Could you check a few things on this model? Use its own coordinates, in mm. Round coordinates to 2 decimals unless told otherwise and drop trailing zeros. Write each loop counter-clockwise with the first axis right and the second up, starting at its lowest first coordinate (ties: lowest second). Pieces come first, ordered by that corner, then holes. Notation, with made-up numbers: M -16,15 L 21,15 A22 ccw 21,34 Z; hole C 32.5,48.25 d4. An arc over 180 degrees is marked long. One line per item, written item: value. Start each with the question number.
(1) If I drill on L1, parallel to Y at x = 24, z = 1.35; L2, parallel to X at y = -45, z = 0.3; L3, parallel to X at y = -21.59, z = 1.25, over which ranges is the centre line in solid material (lowest first)?
(2) I'm going to push a flat-ended pin straight in: pin 1 Ø3 at (x, y) = (20, -47) entering from +Z. Where does the tip first touch, or does it pass through?
(3) Thinking about a two-plate mould opening in X: for faces 1 (the face through (37.3, -51.39, 0.78)), 2 (the face through (-33.027, -62.545, 0.805)), 3 (the face through (12, -40, 1.588)), 4 (the face through (-30.72, -19.87, 0.8)), which applies, released by +X, released by -X, zero draft, split by the parting line, or undercut?
(4) I want a section at A-A on z = 1. Count the separate pieces of the cut face and the enclosed holes in it, and give its area (3 significant figures).
(5) I want a section at C-C on y = -34.29. Please give me the cut outline in (x, z), and give its area (3 significant figures).
(6) I want a section at B-B on x = 41.5. Please give me the cut outline in (y, z).
(7) I want a section at D-D on y = -48.5. Please give me the cut outline in (x, z).
Autodesk Inventor part; units mm, degrees
ref_plane "YZ Plane" through (0, 0, 0) normal (1, 0, 0) x (0, 1, 0)
ref_plane "XZ Plane" through (0, 0, 0) normal (0, 1, 0) x (-1, 0, 0)
ref_plane "XY Plane" through (0, 0, 0) normal (0, 0, 1) x (1, 0, 0)
sketch "Sketch1" plane through (0, 0, 0) normal (0, 0, 1) x (1, 0, 0)
  circle A0 centre (0, 0) radius 63.5
  line L0 (0, 0) -> (63.5, 0)
  line L1 (0, 0) -> (0, -63.5)
  line L2 (0, 0) -> (-127, 0)
  line L3 (-127, 0) -> (-127, -63.5)
  line L4 (-127, -63.5) -> (0, -63.5)
  line L5 (-127, 0) -> (-127, -16.51)
  line L6 (-127, -16.51) -> (61.3161, -16.51)
  dimension "d0" = 127
  dimension "d1" = 127
  dimension "d43" = 16.51
extrude "Extrusion4" add sketch "Sketch1" along normal blind 1.5875 contours L1 L6 A0 | L4 L3 L6 A0 | A0 L6 L1
sketch "Sketch4" plane through (0, 0, 1.5875) normal (0, 0, 1) x (1, 0, 0)
  arc A0 (0, -63.5) -> (61.3161, -16.51) centre (0, 0) ccw
  line L0 (61.3161, -16.51) -> (-59.3339, -16.51)
  line L1 (61.3161, -16.51) -> (-127, -16.51)
  line L2 (-59.3339, -16.51) -> (-59.3339, -62.6422)
  line L3 (-59.3339, -62.6422) -> (-59.3339, -63.5)
  line L4 (-127, -63.5) -> (0, -63.5)
  line L5 (-136.3806, -11.9346) -> (-59.3339, -11.9346)
  line L6 (-59.3339, -11.9346) -> (-59.3339, -68.0966)
  line L7 (-59.3339, -68.0966) -> (-136.3806, -68.0966)
  line L8 (-136.3806, -68.0966) -> (-136.3806, -11.9346)
  point P0 (-59.3339, -16.51)
  dimension "d46" = 120.65
extrude "Extrusion5" cut sketch "Sketch4" against normal blind 1.5875 contours L6 L7 L8 L5 L2 L3
fillet "Fillet2" radius 3.175 1 edges at (61.3161, -16.51, 0.7937)
fillet "Fillet3" radius 3.175 1 edges at (-59.3339, -16.51, 0.7937)
sketch "Sketch5" plane through (0, 0, 1.5875) normal (0, 0, 1) x (1, 0, 0)
  circle A0 centre (-55.6881, -20.1151) radius 2.54
  line L0 (-55.6881, -20.1151) -> (-55.6881, -45.5151)
  line L1 (-55.6881, -45.5151) -> (-55.6881, -58.2151)
  circle A1 centre (-55.6881, -58.2151) radius 2.54
  line L2 (-55.6881, -20.1151) -> (-30.2881, -20.1151)
  line L3 (-55.6881, -58.2151) -> (-30.2881, -58.2151)
  circle A2 centre (-55.6881, -45.5151) radius 2.54
  circle A3 centre (-55.6881, -32.8151) radius 2.54
  line L4 (-59.3339, -13.3218) -> (-33.9321, -13.3218)
  line L5 (-33.9321, -13.3218) -> (-33.9321, -67.3178)
  line L6 (-33.9321, -67.3178) -> (-59.3339, -67.3178)
  line L7 (-59.3339, -67.3178) -> (-59.3339, -13.3218)
  point P0 (0, 0)
  point P1 (-4.8881, -58.2151)
  point P2 (7.8119, -58.2151)
  point P3 (-59.3339, -20.1151)
  point P4 (-42.9881, -20.1151)
  point P5 (-42.9881, -58.2151)
  dimension "d51" = 5.08
  dimension "d52" = 25.4
  dimension "d53" = 12.7
  dimension "d54" = 5.08
  dimension "d55" = 25.4
  dimension "d63" = 25.4
  dimension "d68" = 5.08
  dimension "d69" = 5.08
extrude "Extrusion6" cut sketch "Sketch5" against normal blind 1.5875
sketch "Sketch6" plane through (0, 0, 1.5875) normal (0, 0, 1) x (1, 0, 0)
  line L0 (57.0229, -16.51) -> (-33.9321, -16.51)
  line L1 (-33.9321, -63.5) -> (-33.9321, -16.51)
  line L2 (-33.9321, -21.59) -> (-33.9321, -26.67)
  line L3 (-33.9321, -21.59) -> (-28.8521, -21.59)
  line L4 (-28.8521, -21.59) -> (-28.8521, -16.51)
  circle A0 centre (-28.8521, -21.59) radius 2.54
  line L5 (-28.8521, -21.59) -> (-28.8521, -46.99)
  line L6 (-28.8521, -46.99) -> (-28.8521, -59.69)
  circle A1 centre (-28.8521, -59.69) radius 2.54
  line L7 (-28.8521, -21.59) -> (-3.4521, -21.59)
  line L8 (-3.4521, -21.59) -> (21.9479, -21.59)
  line L9 (21.9479, -21.59) -> (47.3479, -21.59)
  circle A2 centre (-28.8521, -34.29) radius 2.54
  circle A3 centre (-28.8521, -46.99) radius 2.54
  line L10 (-28.8521, -59.69) -> (-3.4521, -59.69)
  line L11 (-3.4521, -59.69) -> (9.2479, -59.69)
  circle A4 centre (47.3479, -21.59) radius 2.54
  line L12 (21.9479, -34.29) -> (21.9479, -46.99)
  circle A5 centre (21.9479, -34.29) radius 2.54
  circle A6 centre (21.9479, -46.99) radius 2.54
  line L13 (21.9479, -34.29) -> (42.2679, -34.29)
  circle A7 centre (42.2679, -34.29) radius 2.54
  line L14 (21.9479, -34.29) -> (33.3071, -44.45)
  circle A8 centre (33.3071, -44.45) radius 2.54
  point P0 (0, 0)
  dimension "d80" = 5.08
  dimension "d81" = 5.08
  dimension "d82" = 5.08
  dimension "d83" = 25.4
  dimension "d84" = 12.7
  dimension "d85" = 5.08
  dimension "d86" = 25.4
  dimension "d87" = 25.4
  dimension "d88" = 25.4
  dimension "d89" = 5.08
  dimension "d90" = 5.08
  dimension "d91" = 25.4
  dimension "d92" = 12.7
  dimension "d96" = 5.08
  dimension "d99" = 5.08
  dimension "d100" = 5.08
  dimension "d101" = 5.08
  dimension "d102" = 20.32
  dimension "d103" = 15.24
  dimension "d104" = 5.08
extrude "Extrusion7" cut sketch "Sketch6" against normal blind 5.08 contours A4 | A1 L10 L6 | L6 L10 A1 | A3 L6 L5 | L5 L6 A3 | A2 L5 | L5 A2 | A0 L7 L4 | L4 L3 A0 | L5 A0 L3 | L7 A0 L5 | L14 A5 L12 | L12 A5 L13 | L13 A5 L14 | A6 | A7 | A8
fillet "Fillet4" radius 3.175 2 edges at (-33.9321, -16.51, 0.7937) (-33.9321, -63.5, 0.7937)
equation "\"d97\" = d93"
properties part number "Sleds"
Found:
1. L1: y = -58.79 to -48.49, -45.49 to -35.79, -32.79 to -16.51
1. L2: x = -33.93 to -30.43, -27.27 to 20.37, 23.53 to 30.83, 35.79 to 44.8
1. L3: x = -33.93 to -31.39, -26.31 to 44.81, 49.89 to 59.72
2. pin 1: stops at z = 1.59
3. face 1: released by +X
3. face 2: released by -X
3. face 3: zero draft
3. face 4: undercut
4. separate pieces: 1
4. enclosed holes: 9
4. area: 3,530 mm²
5. outline: M -33.93,0 L -31.39,0 L -31.39,1.59 L -33.93,1.59 Z; M -26.31,0 L 19.41,0 L 19.41,1.59 L -26.31,1.59 Z; M 24.49,0 L 39.73,0 L 39.73,1.59 L 24.49,1.59 Z; M 44.81,0 L 53.45,0 L 53.45,1.59 L 44.81,1.59 Z
5. area: 115 mm²
6. outline: M -48.06,0 L -36.71,0 L -36.71,1.59 L -48.06,1.59 Z; M -31.87,0 L -16.51,0 L -16.51,1.59 L -31.87,1.59 Z
7. outline: M -33.93,0 L -30.89,0 L -30.89,1.59 L -33.93,1.59 Z; M -26.81,0 L 19.91,0 L 19.91,1.59 L -26.81,1.59 Z; M 23.99,0 L 40.99,0 L 40.99,1.59 L 23.99,1.59 Z
